The model under review builds one solid part; all positions refer to its coordinate system, in mm. Round coordinates to 2 decimals unless told otherwise and drop trailing zeros. Loops run counter-clockwise (first coordinate to the right, second up) from the corner with the lowest first, then second, coordinate; pieces in that order, holes last. Notation, with made-up numbers: (-22.5, 72.5) - (32.5, 72.5) arc R26 cw to (32.5, 106.5) - close; hole circle Ø4 at (78, 46). An arc over 180 degrees is marked (long way). Answer as CSV lines item,"result".
from build123d import *

# Parameters (mm, degrees)
F0_R     = 5.618526
F1_DEPTH = 25.4
F2_R     = 5.08
F3_R     = 3.81
F4_DEPTH = 3


with BuildPart() as f1:
    # F0 (on Top) → F1 (new body)
    with BuildSketch(Plane.XY):
        Circle(F0_R)
    extrude(amount=F1_DEPTH)

    # F2
    f2_edges = [f1.edges().sort_by_distance(p)[0] for p in [
        (-5.618526, 0, 25.4),
    ]]
    fillet(f2_edges, radius=F2_R)

    # F3 (on Top) → F4 (join)
    with BuildSketch(Plane.XY):
        Circle(F3_R)
    extrude(amount=F4_DEPTH)


solid = f1.part
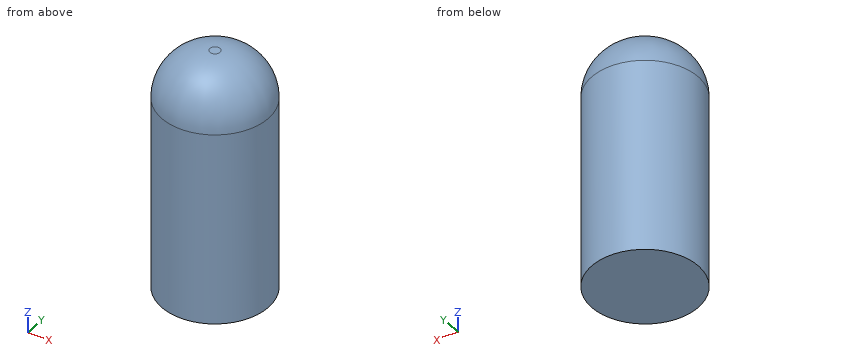
1. Clearance check with flat-ended pins moving along their axes: pin 1 (6 mm diameter, centred on y = 4.5, z = 16, fed in from -X); pin 2 (1.5 mm diameter, centred on x = -0.5, y = -4, fed in from +Z); pin 3 (1 mm diameter, centred on y = 1.5, z = 10.5, fed in from -X). State where each tip first meets the part, or that it passes through.
Numbers:
pin 1,"stops at x = -5.41"
pin 2,"stops at z = 24.6"
pin 3,"stops at x = -5.53"
2. Take a section at A-A (z = 9.75). State the section outline as (x, y) points, plus the area to 3 significant figures.
Numbers:
outline,"circle Ø11.24 at (0, 0)"
area,"99.2 mm²"
3. Wall thickness on probe 1 along X at (y, z) = (-0.25, 11.25); probe 2 along Y at (x, z) = (-2.75, 13.5); probe 3 along Z at (x, y) = (1.5, -1): over which ranges is each line inside the solid? List them lowest first.
Numbers:
probe 1,"x = -5.61 to 5.61"
probe 2,"y = -4.9 to 4.9"
probe 3,"z = 0 to 25.24"
